from build123d import *

# Parameters (mm, degrees)
SKETCH1_W           = 203.2
SKETCH1_H           = 101.6
BOSS_EXTRUDE2_DEPTH = 6.35
SKETCH3_W           = 50.8
SKETCH3_H           = 101.6
BOSS_EXTRUDE3_DEPTH = 50.8
BOSS_EXTRUDE4_DEPTH = 6.35


with BuildPart() as part:
    # Sketch1 → Boss-Extrude2 (new body)
    with BuildSketch(Plane(origin=(0, 0, 0), x_dir=(1, 0, 0), z_dir=(0, 1, 0))):
        with Locations((101.6, 50.8)):
            Rectangle(SKETCH1_W, SKETCH1_H)
    extrude(amount=BOSS_EXTRUDE2_DEPTH)

    # Sketch3 → Boss-Extrude3 (add)
    with BuildSketch(Plane(origin=(0, 6.35, 0), x_dir=(1, 0, 0), z_dir=(0, 1, 0))):
        with Locations((101.6, 50.8)):
            Rectangle(SKETCH3_W, SKETCH3_H)
    extrude(amount=BOSS_EXTRUDE3_DEPTH)

    # Sketch4 → Boss-Extrude4 (add, symmetric)
    with BuildSketch(Plane.XY.offset(-50.8)):
        Polygon((127, 31.75), (152.4, 6.35), (127, 6.35), align=None)
        Polygon((76.2, 31.75), (50.8, 6.35), (76.2, 6.35), align=None)
    extrude(amount=BOSS_EXTRUDE4_DEPTH, both=True)


solid = part.part
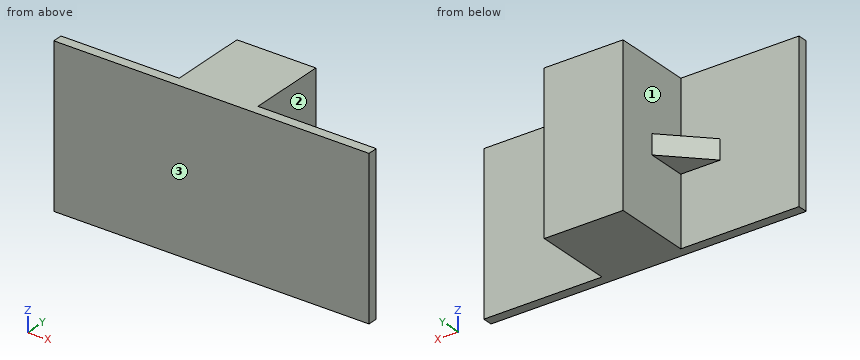
Can you work these out from the model? Positions are in its coordinate system, mm. Face numbers are marked on the shaded views. A direction names the side the tool comes from. Round coordinates to 2 decimals unless told otherwise and drop trailing zeros. Write each loop counter-clockwise with the first axis right and the second up, starting at its lowest first coordinate (ties: lowest second). Pieces come first, ordered by that corner, then holes. Notation, with made-up numbers: (84.5, -10.5) - (141.5, -10.5) arc R18 ccw to (141.5, 11.5) - close; hole circle Ø6 at (19.5, 20.25). An arc over 180 degrees is marked (long way). Write each question's results on one line, items separated by ' | '. Start each with the question number.
1) Suppose I cut it at C-C (x = 129). List the corners of the cut face in (y, z) for me.
2) For pin 1 Ø12 at (x, y) = (55.5, 17) entering from -Z; pin 2 Ø5 at (y, z) = (11, -21.5) entering from +X; pin 3 Ø12 at (y, z) = (25.5, -43.5) entering from -X, each with a flat end and sliding along its axis, tell me the tip position at first contact or that it passes through.
3) Suppose I cut it at B-B (z = -92). List the corners of the cut face in (x, y) for me.
4) Suppose I cut it at D-D (z = -48.5). List the corners of the cut face in (x, y) for me, and give its area (3 significant figures).
5) Please list where these lines run through material, in increasing order: line 1 (X direction, y = 35, z = -7.5); line 2 (Y direction, x = 36.5, z = -73); line 3 (Z direction, x = 73, y = 21).
6) Suppose I cut it at A-A (y = 10). List the corners of the cut face in (x, z) for me.
7) Which directions (+Z, -Z, +X, -X, +Y, -Y) give clear straight access to the entire face, cutting with the end or side of a thin tool? Please do the marked faces 1, 2 and 3.
Here are the results:
1) outline: (0, -101.6) - (6.35, -101.6) - (6.35, -57.15) - (29.75, -57.15) - (29.75, -44.45) - (6.35, -44.45) - (6.35, 0) - (0, 0) - close
2) pin 1: stops at z = -57.15 | pin 2: stops at x = 127 | pin 3: stops at x = 64.03
3) outline: (0, 0) - (203.2, 0) - (203.2, 6.35) - (127, 6.35) - (127, 57.15) - (76.2, 57.15) - (76.2, 6.35) - (0, 6.35) - close
4) outline: (0, 0) - (203.2, 0) - (203.2, 6.35) - (152.4, 6.35) - (127, 31.75) - (127, 57.15) - (76.2, 57.15) - (76.2, 31.75) - (50.8, 6.35) - (0, 6.35) - close | area: 4,520 mm2
5) line 1: x = 76.2 to 127 | line 2: y = 0 to 6.35 | line 3: z = -57.15 to -44.45
6) outline: (54.45, -57.15) - (76.2, -57.15) - (76.2, -101.6) - (127, -101.6) - (127, -57.15) - (148.75, -57.15) - (148.75, -44.45) - (127, -44.45) - (127, 0) - (76.2, 0) - (76.2, -44.45) - (54.45, -44.45) - close
7) face 1: -X, +Y | face 2: +X, +Y | face 3: +Z, -Z, +X, -X, -Y
